Work out the finished part from the listing and answer in its coordinate system (mm). Coordinates: 2 decimals unless noted, no trailing zeros. Order: outer loops, then holes, each group sorted by start corner. A loop starts at its lowest first (then second) coordinate and runs counter-clockwise, first axis right, second up. Notation, with made-up numbers: (-8.75, 32) -> (46.25, 32) arc R31 cw to (46.25, 65) -> close; hole circle Ø4 at (-13.75, 88). An arc over 180 degrees is marked (long way). Answer as CSV lines item,"result". Start each with the question number.
Item 1: Section C-C (z = 43) is taken. Write down the section's boundary in (x, y).
Item 2: Straight lines are drawn through the part: L1, parallel to Z at x = 2.75, y = 10.75; L2, parallel to Y at x = -7.25, z = 53; L3, parallel to Z at x = -10.25, y = -1. For each, find the intervals that lie inside material, in ascending order.
Item 3: Each of these flat-tipped pins is pushed along its axis until it touches: pin 1 Ø5 at (x, z) = (8, 10.5) entering from +Y; pin 2 Ø5 at (x, z) = (-7.5, 51.5) entering from +Y; pin 3 Ø6 at (x, z) = (-0.5, 31) entering from -Y; pin 4 Ø3 at (x, z) = (8, 29.5) entering from +Y. Where does it stop, or does it pass through?
Item 4: Section D-D (z = 32) is taken. Write down the section's boundary in (x, y), then the cut area to 3 significant figures.
Item 5: Section A-A (y = 0) is taken. Write down the section's boundary in (x, z), then the cut area to 3 significant figures.
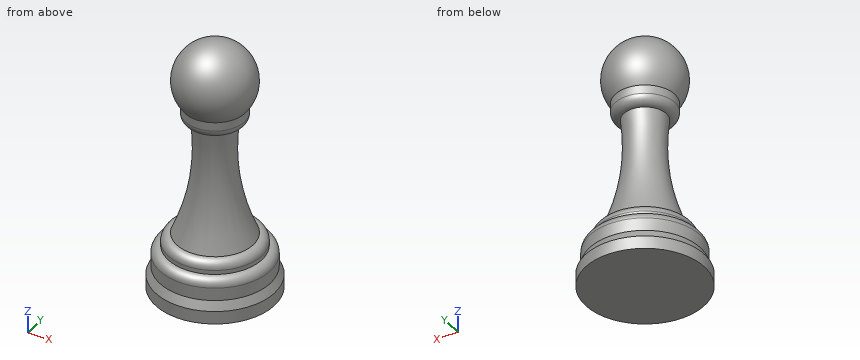
Solid Edge part; units mm, degrees
sketch "Sketch1" plane through (0, 0, 0) normal (0, -1, 0) x (1, 0, 0)
  arc A0 (11, 10.9653) -> (9, 12.9653) centre (9, 10.9653) ccw
  line L0 (11, 10) -> (11, 10.9653)
  arc A1 (13, 8) -> (11, 10) centre (11, 8) ccw
  line L1 (13, 5) -> (13, 8)
  line L2 (13, 5) -> (14, 3)
  line L3 (14, 0) -> (14, 3)
  line L4 (0, 0) -> (14, 0)
  line L5 (0, 0) -> (0, 59)
  line L6 (7, 42) -> (7, 44)
  arc A2 (5, 40) -> (7, 42) centre (5, 42) ccw
  arc A3 (5, 40) -> (9, 12.9653) centre (54.5786, 33.5223) ccw
  arc A4 (0, 58.6569) -> (7, 44) centre (0, 49.6569) cw
revolve "RevolvedProtrusion1" add sketch "Sketch1" angle 360 about axis through (0, 0, 0) along (0, 0, 1)
Checked values:
1,outline,"circle Ø14 at (0, 0)"
2,L1,"z = 0 to 10"
2,L2,"y = -4.15 to 4.15"
2,L3,"z = 0 to 12.49"
3,pin 1,"stops at y = 11.25"
3,pin 2,"stops at y = 7.33"
3,pin 3,"stops at y = -4.88"
3,pin 4,"passes through"
4,outline,"circle Ø9.2 at (0, 0)"
4,area,"66.5 mm^2"
5,outline,"(-14, 0) -> (14, 0) -> (14, 3) -> (13, 5) -> (13, 8) arc R2 ccw to (11, 10) -> (11, 10.97) arc R2 ccw to (9, 12.97) arc R50 cw to (5, 40) arc R2 ccw to (7, 42) -> (7, 44) arc R9 ccw (long way) to (-7, 44) -> (-7, 42) arc R2 ccw to (-5, 40) arc R50 cw to (-9, 12.97) arc R2 ccw to (-11, 10.97) -> (-11, 10) arc R2 ccw to (-13, 8) -> (-13, 5) -> (-14, 3) -> close"
5,area,"915 mm^2"
